Geometry: final body of the model. Coordinates: model frame, mm. A direction names the side the tool comes from. Give positions to 0.01 mm unless a question says otherwise; leave off trailing zeros. Write each loop counter-clockwise with the first axis right and the second up, starting at its lowest first coordinate (ties: lowest second). Pieces come first, ordered by that corner, then holes.
```python
from build123d import *

# Parameters (mm, degrees)
ESQUISSE1_R                  = 200
ESQUISSE1_R_2                = 150
BOSS_EXTRU_1_DEPTH           = 20
TROU_TARAUD_M161_D           = 14
ENL_V_MAT_EXTRU_3_DEPTH      = 2
R_P_TITION_CIRCULAIRE1_COUNT = 2
R_P_TITION_CIRCULAIRE1_ANGLE = 70
R_P_TITION_CIRCULAIRE2_COUNT = 2
R_P_TITION_CIRCULAIRE2_ANGLE = 110


with BuildPart() as part:
    # Esquisse1 → Boss.-Extru.1 (new body)
    with BuildSketch(Plane(origin=(0, 0, 0), x_dir=(1, 0, 0), z_dir=(0, 1, 0))):
        with Locations(Location((0, 0, 0), (0, 0, 270))):  # turned: the seam where the file's is
            Circle(ESQUISSE1_R)
        with Locations(Location((0, 0, 0), (0, 0, 270))):  # turned: the seam where the file's is
            Circle(ESQUISSE1_R_2, mode=Mode.SUBTRACT)
    extrude(amount=BOSS_EXTRU_1_DEPTH)

    # Trou taraud_ M161 (through all)
    with Locations(Plane(origin=(0, 20, 0), x_dir=(1, 0, 0), z_dir=(0, 1, 0))):
        with Locations((112.487831695, 134.057777546)):
            trou_taraud_m161 = Hole(TROU_TARAUD_M161_D / 2)

    # Esquisse4 → Enl_v. mat.-Extru.3 (cut)
    with BuildSketch(Plane(origin=(0, 20, 0), x_dir=(1, 0, 0), z_dir=(0, 1, 0))):
        Polygon((-11.490666647, 9.641814145), (11.490666647, -9.641814145), (140.048188584, 143.567074478), (117.066855291, 162.850702769), align=None)
    enl_v_mat_extru_3 = extrude(amount=-ENL_V_MAT_EXTRU_3_DEPTH, mode=Mode.SUBTRACT)

    # R_p_tition circulaire1: Trou taraud_ M161, Enl_v. mat.-Extru.3 ×2 about axis
    r_p_tition_circulaire1_axis = Axis((0, 0, 0), (0, -1, 0))
    add([trou_taraud_m161.rotate(r_p_tition_circulaire1_axis, i * R_P_TITION_CIRCULAIRE1_ANGLE / (R_P_TITION_CIRCULAIRE1_COUNT - 1)) for i in range(1, R_P_TITION_CIRCULAIRE1_COUNT)], mode=Mode.SUBTRACT)
    add([enl_v_mat_extru_3.rotate(r_p_tition_circulaire1_axis, i * R_P_TITION_CIRCULAIRE1_ANGLE / (R_P_TITION_CIRCULAIRE1_COUNT - 1)) for i in range(1, R_P_TITION_CIRCULAIRE1_COUNT)], mode=Mode.SUBTRACT)

    # R_p_tition circulaire2: Trou taraud_ M161, Enl_v. mat.-Extru.3 ×2 about axis
    r_p_tition_circulaire2_axis = Axis((0, 0, 0), (0, -1, 0))
    add([trou_taraud_m161.rotate(r_p_tition_circulaire2_axis, i * R_P_TITION_CIRCULAIRE2_ANGLE / (R_P_TITION_CIRCULAIRE2_COUNT - 1)) for i in range(1, R_P_TITION_CIRCULAIRE2_COUNT)], mode=Mode.SUBTRACT)
    add([enl_v_mat_extru_3.rotate(r_p_tition_circulaire2_axis, i * R_P_TITION_CIRCULAIRE2_ANGLE / (R_P_TITION_CIRCULAIRE2_COUNT - 1)) for i in range(1, R_P_TITION_CIRCULAIRE2_COUNT)], mode=Mode.SUBTRACT)


solid = part.part
```
Item 1: Section C-C, the plane y = 7. Return the cut outline in (x, z).
Found:
outline: circle Ø400 at (0, 0); hole circle Ø300 at (0, 0); hole circle Ø14 at (87.5, 151.55); hole circle Ø14 at (112.49, -134.06); hole circle Ø14 at (164.45, 59.85)
Item 2: Section B-B, the plane x = -116. Return the cut outline in (y, z).
Found:
outline: (0, -162.92) - (20, -162.92) - (20, -95.1) - (0, -95.1) - close; (0, 95.1) - (20, 95.1) - (20, 162.92) - (0, 162.92) - close
Item 3: Line query: L1, parallel to Z at x = 0, y = 9.5; L2, parallel to X at y = 6.75, z = 127. Output: solid intervals per line, ascending.
Found:
L1: z = -200 to -150, 150 to 200
L2: x = -154.5 to -79.82, 79.82 to 154.5
Item 4: Pin query (flat end, axial travel): pin 1 Ø1.5 at (x, y) = (126.5, 13.5) entering from -Z; pin 2 Ø2 at (x, y) = (-64, 10.5) entering from -Z; pin 3 Ø8 at (x, y) = (53.5, 7.5) entering from -Z. Return the tip coordinate at first contact, or that it passes through.
Found:
pin 1: stops at z = -155.52
pin 2: stops at z = -189.82
pin 3: stops at z = -193.78
Item 5: Section A-A, the plane z = 0. Return the cut outline in (x, y).
Found:
outline: (-200, 0) - (-150, 0) - (-150, 20) - (-200, 20) - close; (150, 0) - (200, 0) - (200, 20) - (150, 20) - close
Item 6: Pull-direction query (Z, two-part tool) for faces 4 (the face through (-76.6, 9.86, 184.75)), 5 (the face through (100.8, 19.014, -143.465)), 6 (the face through (136, 20, 114)); classes: +Z half, -Z half, draft (parallel to the pull), parting line (faces both ways), or undercut.
Found:
face 4: parting line
face 5: undercut
face 6: draft
Item 7: Reachability of faces 1 (the face through (100.34, 19.01, 143.79)), 2 (the face through (158.368, 19.014, 73.604)), 3 (the face through (118, 18, -140)) from +Z, -Z, +X, -X, +Y, -Y: full face, straight path, thin tool, end or side. Return the list, or none.
Found:
face 1: +Z, +Y
face 2: +X, +Y
face 3: +Y
